from build123d import *

# Parameters (mm, degrees)
F0_W     = 44.2640645027
F0_H     = 38.2859354973
F1_DEPTH = 6.35


with BuildPart() as f1:
    # F0 (on Front) → F1 (new body)
    with BuildSketch(Plane.XZ):
        Polygon((41.275, -41.275), (41.275, 41.275), (22.1320322514, 41.275), (-22.1320322514, 41.275), (-41.275, 41.275), (-41.275, -41.275), (-15.875, -41.275), (-7.8206129843, -41.275), (7.8206129843, -41.275), (15.875, -41.275), align=None)
        with Locations((0, 60.4179677486)):
            Rectangle(F0_W, F0_H)
        Polygon((15.875, -85.725), (15.875, -41.275), (7.8206129843, -41.275), (7.8206129843, -85.5907460871), (7.8206129843, -85.725), align=None)
        Polygon((-7.8206129843, -85.5907460871), (-7.8206129843, -41.275), (-15.875, -41.275), (-15.875, -85.725), (-7.8206129843, -85.725), align=None)
    extrude(amount=F1_DEPTH)


solid = f1.part
Can you work these out from the model? Positions are in its coordinate system, mm. A direction names the side the tool comes from. Round coordinates to 2 decimals unless told otherwise and drop trailing zeros. Loops run counter-clockwise (first coordinate to the right, second up) from the corner with the lowest first, then second, coordinate; pieces in that order, holes last. Notation, with made-up numbers: (-20, 68) - (-6, 68) arc R12 ccw to (-6, 72) - close; hole circle Ø9 at (78, 26). An arc over 180 degrees is marked (long way). Answer in a Markdown table with one row per item. Add a question column.
Q1. I want a section at C-C on x = 19. List the corners of the cut face in (y, z) for me (3 decimals), and give its area (3 significant figures).
Q2. We'd pull the mould along X, two halves only. Please class faces 1 (the flat face through (-15.875, -3, -63)), 2 (the flat face through (0, -3, -41.275)), 3 (the flat face through (22.132, -3, 60)), 4 (the flat face through (-7.821, -3, -64)): pulls with the +X half, pulls with the -X half, needs draft (parallel to the pull), parting line crosses it, or undercut.
Q3. Which directions (+Z, -Z, +X, -X, +Y, -Y) give clear straight access to the entire face, cutting with the end or side of a thin tool? Please do faces 5 (the flat face through (-22.132, -3, 60)), 6 (the flat face through (15.875, -3, -64)), 7 (the flat face through (7.821, -3, -63)), 8 (the flat face through (32, -3, 41.275)), 9 (the flat face through (-29, -3, -41.275)).
Q4. I need wall thicknesses on L1, parallel to X at y = -5.25, z = -57.5 (3 decimals); L2, parallel to X at y = -3.5, z = 71; L3, parallel to Z at x = -23, y = -0.75 (3 decimals). Which ranges of each line are inside material? Lowest first, please.
Q5. I want a section at D-D on z = 62. List the corners of the cut face in (x, y) for me, and give its area (3 significant figures).
Q6. For pin 1 Ø3 at (y, z) = (-4.5, -69) entering from -X (3 decimals); pin 2 Ø3 at (x, y) = (-33, -2.5) entering from -Z (3 decimals); pin 3 Ø3 at (y, z) = (-2.5, 68) entering from +X; pin 4 Ø10 at (x, z) = (32.5, -9) entering from +Y, each with a flat end and sliding along its axis, tell me the tip position at first contact or that it passes through.
Q7. I want a section at A-A on z = -56. List the corners of the cut face in (x, y) for me (3 decimals).
Q8. I want a section at B-B on y = -2.75. List the corners of the cut face in (x, z) for me (3 decimals), and give its area (3 significant figures).
A:
| question | item | result |
|---|---|---|
| 1 | outline | (-6.35, -41.275) - (0, -41.275) - (0, 79.561) - (-6.35, 79.561) - close |
| 1 | area | 767 mm^2 |
| 2 | face 1 | pulls with the -X half |
| 2 | face 2 | undercut |
| 2 | face 3 | pulls with the +X half |
| 2 | face 4 | undercut |
| 3 | face 5 | +Z, -X, +Y, -Y |
| 3 | face 6 | -Z, +X, +Y, -Y |
| 3 | face 7 | -Z, +Y, -Y |
| 3 | face 8 | +Z, +X, +Y, -Y |
| 3 | face 9 | -Z, -X, +Y, -Y |
| 4 | L1 | -15.875 to -7.821, 7.821 to 15.875 |
| 4 | L2 | -22.13 to 22.13 |
| 4 | L3 | -41.275 to 41.275 |
| 5 | outline | (-22.13, -6.35) - (22.13, -6.35) - (22.13, 0) - (-22.13, 0) - close |
| 5 | area | 281 mm^2 |
| 6 | pin 1 | x = -15.875 |
| 6 | pin 2 | z = -41.275 |
| 6 | pin 3 | x = 22.13 |
| 6 | pin 4 | y = 0 |
| 7 | outline | (-15.875, -6.35) - (-7.821, -6.35) - (-7.821, 0) - (-15.875, 0) - close; (7.821, -6.35) - (15.875, -6.35) - (15.875, 0) - (7.821, 0) - close |
| 8 | outline | (-41.275, -41.275) - (-15.875, -41.275) - (-15.875, -85.725) - (-7.821, -85.725) - (-7.821, -41.275) - (7.821, -41.275) - (7.821, -85.725) - (15.875, -85.725) - (15.875, -41.275) - (41.275, -41.275) - (41.275, 41.275) - (22.132, 41.275) - (22.132, 79.561) - (-22.132, 79.561) - (-22.132, 41.275) - (-41.275, 41.275) - close |
| 8 | area | 9,230 mm^2 |
